For this review, take the finished solid that the model builds, in its own axes (mm). A direction names the side the tool comes from. Round coordinates to 2 decimals unless told otherwise and drop trailing zeros. Order: outer loops, then holes, each group sorted by start corner. A loop starts at its lowest first (then second) coordinate and runs counter-clockwise, first axis right, second up. Notation, with made-up numbers: (8.5, -2.75) -> (55.5, -2.75) arc R36 cw to (55.5, 31.25) -> close; hole circle Ø8 at (83.25, -39.75). An arc over 180 degrees is marked (long way). Answer in a Markdown table with one row per item.
```python
from build123d import *

# Parameters (mm, degrees)
BOSS_EXTRUDE1_DEPTH     = 23
CUT_EXTRUDE1_REACH      = 39.885
CUT_EXTRUDE2_REACH      = 35.693
SKETCH3_R               = 2.25
CUT_EXTRUDE3_START      = 23
SKETCH4_R               = 3.55
CUT_EXTRUDE3_DEPTH      = 13
FILLET1_R               = 2
CHAMFER1_SIZE           = 13
CHAMFER2_SIZE           = 1
CUT_EXTRUDE4_REACH      = 35.693
CUT_EXTRUDE4_END_RADIUS = 12.5
SKETCH5_R               = 3
CHAMFER3_SIZE           = 1


with BuildPart() as part:
    # Sketch1 → Boss-Extrude1 (new body)
    with BuildSketch(Plane(origin=(0, 0, 0), x_dir=(1, 0, 0), z_dir=(0, 1, 0))):
        Polygon((0, 10), (-22.5, 10), (-22.5, -10), (22.5, -10), (22.5, 10), align=None)
    extrude(amount=BOSS_EXTRUDE1_DEPTH)

    # Sketch2 → Cut-Extrude1 (cut, up to next)
    with BuildSketch(Plane.XY.offset(10), mode=Mode.PRIVATE) as cut_extrude1_sk1:
        with BuildLine():
            Line((-12.5, 0), (-22.5, 0))
            Line((-22.5, 0), (-22.5, -2.522641864))
            Line((-22.5, -2.522641864), (22.5, -2.522641864))
            Line((22.5, -2.522641864), (22.5, 0))
            Line((22.5, 0), (12.5, 0))
            ThreePointArc((12.5, 0), (0, 12.5), (-12.5, 0))
        make_face()
    cut_extrude1_tool1 = extrude(cut_extrude1_sk1.sketch, amount=-CUT_EXTRUDE1_REACH, mode=Mode.PRIVATE) & part.part
    add(cut_extrude1_tool1.solids().sort_by_distance((0, 3.22853, 10))[0], mode=Mode.SUBTRACT)

    # Sketch3 → Cut-Extrude2 (cut, up to next)
    with BuildSketch(Plane(origin=(0, 0, 0), x_dir=(1, 0, 0), z_dir=(0, 1, 0)), mode=Mode.PRIVATE) as cut_extrude2_sk1:
        with Locations(Location((-17.5, -5, 0), (0, 0, 270))):
            Circle(SKETCH3_R)
    cut_extrude2_tool1 = extrude(cut_extrude2_sk1.sketch, amount=CUT_EXTRUDE2_REACH, mode=Mode.PRIVATE) & part.part
    # Sketch3 → Cut-Extrude2 (cut, up to next)
    with BuildSketch(Plane(origin=(0, 0, 0), x_dir=(1, 0, 0), z_dir=(0, 1, 0)), mode=Mode.PRIVATE) as cut_extrude2_sk2:
        with Locations(Location((-17.5, 5, 0), (0, 0, 270))):
            Circle(SKETCH3_R)
    cut_extrude2_tool2 = extrude(cut_extrude2_sk2.sketch, amount=CUT_EXTRUDE2_REACH, mode=Mode.PRIVATE) & part.part
    cut_extrude2_1 = cut_extrude2_tool1.solids().sort_by_distance((-17.5, 0, 5))[0]
    add(cut_extrude2_1, mode=Mode.SUBTRACT)
    cut_extrude2_2 = cut_extrude2_tool2.solids().sort_by_distance((-17.5, 0, -5))[0]
    add(cut_extrude2_2, mode=Mode.SUBTRACT)
    cut_extrude2 = cut_extrude2_1 + cut_extrude2_2  # Cut-Extrude2 as one shape, for the pattern or mirror that repeats it

    # Mirror1: Cut-Extrude2 across plane
    add(cut_extrude2.mirror(Plane(origin=(0, 0, 0), x_dir=(0, 0, 1), z_dir=(1, 0, 0))), mode=Mode.SUBTRACT)

    # Sketch4 → Cut-Extrude3 (cut)
    with BuildSketch(Plane(origin=(0, 0, 0), x_dir=(1, 0, 0), z_dir=(0, 1, 0)).offset(CUT_EXTRUDE3_START)):
        with Locations(Location((-17.5, 5, 0), (0, 0, 270))):
            Circle(SKETCH4_R)
        with Locations(Location((-17.5, -5, 0), (0, 0, 270))):
            Circle(SKETCH4_R)
    cut_extrude3 = extrude(amount=-CUT_EXTRUDE3_DEPTH, mode=Mode.SUBTRACT)

    # Mirror2: Cut-Extrude3 across plane
    add(cut_extrude3.mirror(Plane(origin=(0, 0, 0), x_dir=(0, 0, 1), z_dir=(1, 0, 0))), mode=Mode.SUBTRACT)

    # Fillet1
    fillet1_edges = [part.edges().sort_by_distance(p)[0] for p in [
        (0, 12.5, 10),
        (0, 12.5, -10),
    ]]
    fillet(fillet1_edges, radius=FILLET1_R)

    # Chamfer1
    # the kernel refuses this chamfer: 13 mm, written as the material it takes off along each edge
    with BuildSketch(Plane(origin=(-22.5, 23, -43.431878844), x_dir=(0.9996219169112968, 0.027495876610586424, 0), z_dir=(0, 0, 1))) as chamfer1_piece_1:
        Polygon((CHAMFER1_SIZE * 0.999621916911, -CHAMFER1_SIZE * 0.0274958766106), (-CHAMFER1_SIZE * 0.0274958766106, -CHAMFER1_SIZE * 0.999621916911), (0, 0), align=None)
    extrude(amount=86.863757687, mode=Mode.SUBTRACT)
    with BuildSketch(Plane(origin=(22.5, 23, 43.431878844), x_dir=(0.027495876610586424, -0.9996219169112968, 0), z_dir=(0, 0, -1))) as chamfer1_piece_2:
        Polygon((CHAMFER1_SIZE * 0.999621916911, CHAMFER1_SIZE * 0.0274958766106), (-CHAMFER1_SIZE * 0.0274958766106, CHAMFER1_SIZE * 0.999621916911), (0, 0), align=None)
    extrude(amount=86.863757687, mode=Mode.SUBTRACT)

    # Chamfer2
    chamfer2_edges = [part.edges().sort_by_distance(p)[0] for p in [
        (0, 23, -10),
        (0, 23, 10),
        (-22.5, 5, -10),
        (22.5, 5, -10),
        (-16, 16.5, -10),
        (16, 16.5, -10),
        (22.5, 5, 10),
        (-22.5, 5, 10),
        (-16, 16.5, 10),
        (16, 16.5, 10),
    ]]
    chamfer(chamfer2_edges, length=CHAMFER2_SIZE)

    # Cut-Extrude4: up to this cylinder (the profile starts outside it)
    cut_extrude4_end = Plane(origin=(0, 0, 0), z_dir=(0, 0, 1)) * Cylinder(CUT_EXTRUDE4_END_RADIUS, 97.386, mode=Mode.PRIVATE)
    # Sketch5 → Cut-Extrude4 (cut, up to the surface)
    with BuildSketch(Plane(origin=(0, 23, 0), x_dir=(1, 0, 0), z_dir=(0, 1, 0)), mode=Mode.PRIVATE) as cut_extrude4_sk1:
        with Locations(Location((0, 0, 0), (0, 0, 270))):
            Circle(SKETCH5_R)
    cut_extrude4_tool1 = extrude(cut_extrude4_sk1.sketch, amount=-CUT_EXTRUDE4_REACH, mode=Mode.PRIVATE) - cut_extrude4_end
    add(cut_extrude4_tool1.solids().sort_by_distance((0, 23, 0))[0], mode=Mode.SUBTRACT)

    # Chamfer3
    chamfer3_edges = [part.edges().sort_by_distance(p)[0] for p in [
        (0, 23, -3),
    ]]
    chamfer(chamfer3_edges, length=CHAMFER3_SIZE)


solid = part.part
```
Q1. Clearance check with flat-ended pins moving along their axes: pin 1 Ø7 at (x, z) = (-17.5, -5) entering from +Y; pin 2 Ø5 at (x, z) = (4, 5) entering from -Y; pin 3 Ø8 at (x, z) = (18, -6.5) entering from +Y. State where each tip first meets the part, or that it passes through.
Answer key:
| item | result |
|---|---|
| pin 1 | stops at y = 10 |
| pin 2 | stops at y = 10.68 |
| pin 3 | stops at y = 18.5 |
Q2. Take a section at B-B, the plane z = -5. Write out the cut boundary in (x, y).
Answer key:
| item | result |
|---|---|
| outline | (-22.5, 0) -> (-19.75, 0) -> (-19.75, 10) -> (-21.05, 10) -> (-21.05, 11.45) -> (-22.5, 10) -> close; (-15.25, 0) -> (-12.5, 0) arc R12.5 cw to (12.5, 0) -> (15.25, 0) -> (15.25, 10) -> (13.95, 10) -> (13.95, 18.55) -> (9.5, 23) -> (-9.5, 23) -> (-13.95, 18.55) -> (-13.95, 10) -> (-15.25, 10) -> close; (19.75, 0) -> (22.5, 0) -> (22.5, 10) -> (21.05, 11.45) -> (21.05, 10) -> (19.75, 10) -> close |
Q3. To check wall thickness, follow probe 1 along Z at (x, y) = (17.5, 12); probe 2 along X at (y, z) = (10.25, 8); probe 3 along X at (y, z) = (11.5, 7.75) (3 decimals). State the ranges of each line that lie inside material, in increasing order.
Answer key:
| item | result |
|---|---|
| probe 1 | z = -10 to -8.55, -1.45 to 1.45, 8.55 to 10 |
| probe 2 | x = -22.25 to -19.4, -15.6 to -7.15, 7.15 to 15.6, 19.4 to 22.25 |
| probe 3 | x = -21 to -19.745, -15.255 to -4.899, 4.899 to 15.255, 19.745 to 21 |
Q4. Take a section at A-A, the plane z = 0. Write out the cut boundary in (x, y).
Answer key:
| item | result |
|---|---|
| outline | (-22.5, 0) -> (-12.5, 0) arc R12.5 cw to (-3, 12.13) -> (-3, 22) -> (-4, 23) -> (-9.5, 23) -> (-22.5, 10) -> close; (3, 12.13) arc R12.5 cw to (12.5, 0) -> (22.5, 0) -> (22.5, 10) -> (9.5, 23) -> (4, 23) -> (3, 22) -> close |
Q5. Take a section at D-D, the plane y = 15.5. Write out the cut boundary in (x, z).
Answer key:
| item | result |
|---|---|
| outline | (-17, -9) -> (-15.59, -10) -> (15.59, -10) -> (17, -9) -> (17, -8.51) arc R3.55 cw to (17, -1.49) -> (17, 1.49) arc R3.55 cw to (17, 8.51) -> (17, 9) -> (15.59, 10) -> (-15.59, 10) -> (-17, 9) -> (-17, 8.51) arc R3.55 cw to (-17, 1.49) -> (-17, -1.49) arc R3.55 cw to (-17, -8.51) -> close; hole circle Ø6 at (0, 0) |
Q6. Take a section at C-C, the plane x = 17.5. Write out the cut boundary in (y, z).
Answer key:
| item | result |
|---|---|
| outline | (0, -10) -> (13.59, -10) -> (15, -9) -> (15, -8.55) -> (10, -8.55) -> (10, -7.25) -> (0, -7.25) -> close; (0, -2.75) -> (10, -2.75) -> (10, -1.45) -> (15, -1.45) -> (15, 1.45) -> (10, 1.45) -> (10, 2.75) -> (0, 2.75) -> close; (0, 7.25) -> (10, 7.25) -> (10, 8.55) -> (15, 8.55) -> (15, 9) -> (13.59, 10) -> (0, 10) -> close |
Q7. Tool access review of faces 4 (the face through (-13.98, 13.42, 4.54)), 5 (the face through (0.1, 22.5, -9.5)): name each direction out of +Z, -Z, +X, -X, +Y, -Y from which nothing blocks a thin tool from reaching the whole face with its end or side.
Answer key:
| item | result |
|---|---|
| face 4 | +Y |
| face 5 | -Z, +X, -X, +Y |
Q8. The part is to be moulded in two halves that separate along X. For faces 1 (the face through (-18, 0, 0)), 2 (the face through (20, 10, 5)), 3 (the face through (22, 4.9, -9.5)), say which applies: +X half, -X half, draft (parallel to the pull), parting line (faces both ways), or undercut.
Answer key:
| item | result |
|---|---|
| face 1 | draft |
| face 2 | undercut |
| face 3 | +X half |
